For this review, take the finished solid that the model builds, in its own axes (mm). A direction names the side the tool comes from. Coordinates: 2 decimals unless noted, no trailing zeros. Order: outer loops, then holes, each group sorted by start corner. A loop starts at its lowest first (then second) coordinate and runs counter-clockwise, first axis right, second up. Notation, with made-up numbers: (60, 76.5) - (72, 76.5) arc R29 ccw to (72, 106.5) - close; hole circle Ø7 at (6.5, 68). An arc over 180 degrees is marked (long way). One line per item, written item: value. Start each with the question number.
(1) Consider section A-A on x = 0. Write out the cut boundary in (y, z), then the cut area to 3 significant figures.
(2) Consider section B-B on y = -14.5. Write out the cut boundary in (x, z), then the cut area to 3 significant figures.
(3) Consider section C-C on z = 0. Write out the cut boundary in (x, y), then the cut area to 3 significant figures.
(4) To check wall thickness, follow line 1 along Z through (x, y) = (0, -13); line 2 along Y through (x, z) = (6.5, 8); line 3 along X through (y, z) = (-24, 2). State the ranges of each line that lie inside material, in increasing order.
(5) For faces 4 (the cylindrical face through (10.316, -17.748, -7.91)), 5 (the flat face through (-8, 0, 11)), list the 3-axis set-ups (+Z, -Z, +X, -X, +Y, -Y) from which the entire face can be reached by the end or side of a thin tool; tool diameter is ignored.
(6) Mouldability with a two-part tool opening along Z and no side actions: class faces 1 (the flat face through (0, -223, 0)), 2 (the flat face through (0, -110, -25)), 3 (the flat face through (0, -36, 0)) as released by +Z, released by -Z, zero draft, split by the parting line, or undercut.
```python
from build123d import *

# Parameters (mm, degrees)
F0_W     = 65
F0_H     = 50
F1_DEPTH = 223
F3_R     = 13
F4_DEPTH = 36


with BuildPart() as f1:
    # F0 (on Front) → F1 (new body)
    with BuildSketch(Plane.XZ):
        Rectangle(F0_W, F0_H)
    extrude(amount=F1_DEPTH)

    # F3 (on face) → F4 (cut)
    with BuildSketch(Plane(origin=(0, 0, 0), x_dir=(-1, 0, 0), z_dir=(0, 1, 0))):
        Circle(F3_R)
    extrude(amount=-F4_DEPTH, mode=Mode.SUBTRACT)


solid = f1.part
```
Geometry check:
1. outline: (-223, -25) - (0, -25) - (0, -13) - (-36, -13) - (-36, 13) - (0, 13) - (0, 25) - (-223, 25) - close
1. area: 10,200 mm^2
2. outline: (-32.5, -25) - (32.5, -25) - (32.5, 25) - (-32.5, 25) - close; hole circle Ø26 at (0, 0)
2. area: 2,720 mm^2
3. outline: (-32.5, -223) - (32.5, -223) - (32.5, 0) - (13, 0) - (13, -36) - (-13, -36) - (-13, 0) - (-32.5, 0) - close
3. area: 13,600 mm^2
4. line 1: z = -25 to -13, 13 to 25
4. line 2: y = -223 to -36
4. line 3: x = -32.5 to -12.85, 12.85 to 32.5
5. face 4: +Y
5. face 5: +Z, -Z, +X, -X, +Y
6. face 1: zero draft
6. face 2: released by -Z
6. face 3: undercut
